CAD build for the part. Positions are in the model's coordinates, mm. Give positions to 0.01 mm unless a question says otherwise; leave off trailing zeros. Write each loop counter-clockwise with the first axis right and the second up, starting at its lowest first coordinate (ties: lowest second). Pieces come first, ordered by that corner, then holes. Notation, with made-up numbers: (-16.75, 25.25) -> (37.25, 25.25) arc R20 ccw to (37.25, 60.25) -> close; hole circle Ø6 at (29.25, 84). An arc over 180 degrees is marked (long way). Answer as a JSON object with one key per item and string values.
```python
from build123d import *

# Parameters (mm, degrees)
ESQUISSE1_R             = 71.6
ESQUISSE1_R_2           = 33.05
BOSS_EXTRU_1_DEPTH      = 5
ESQUISSE2_R             = 6.5
ENL_V_MAT_EXTRU_1_DEPTH = 6
ESQUISSE3_R             = 3.1
ENL_V_MAT_EXTRU_2_DEPTH = 6
CHANFREIN1_SIZE         = 4


with BuildPart() as part:
    # Esquisse1 → Boss.-Extru.1 (new body)
    with BuildSketch(Plane.XY):
        Circle(ESQUISSE1_R)
        Circle(ESQUISSE1_R_2, mode=Mode.SUBTRACT)
    extrude(amount=BOSS_EXTRU_1_DEPTH)

    # Esquisse2 → Enlèv. mat.-Extru.1 (cut, through all)
    with BuildSketch(Plane.XY.offset(5)):
        with Locations((0, 54)):
            Circle(ESQUISSE2_R)
        with Locations((54, 0)):
            Circle(ESQUISSE2_R)
        with Locations((-54, 0)):
            Circle(ESQUISSE2_R)
        with Locations((0, -54)):
            Circle(ESQUISSE2_R)
    extrude(amount=-ENL_V_MAT_EXTRU_1_DEPTH, mode=Mode.SUBTRACT)

    # Esquisse3 → Enlèv. mat.-Extru.2 (cut, through all)
    with BuildSketch(Plane.XY.offset(5)):
        with Locations((-38.183766184, 38.183766184)):
            Circle(ESQUISSE3_R)
        with Locations((38.183766184, -38.183766184)):
            Circle(ESQUISSE3_R)
    extrude(amount=-ENL_V_MAT_EXTRU_2_DEPTH, mode=Mode.SUBTRACT)

    # Chanfrein1
    chanfrein1_edges = [part.edges().sort_by_distance(p)[0] for p in [
        (-41.283766184, 38.183766184, 5),
        (35.083766184, -38.183766184, 5),
    ]]
    chamfer(chanfrein1_edges, length=CHANFREIN1_SIZE)


solid = part.part
```
1) Slice it at C-C (y = 54). List the corners of the cut face in (x, z).
Model answer:
{"outline": "(-47.02, 0) -> (-6.5, 0) -> (-6.5, 5) -> (-47.02, 5) -> close; (6.5, 0) -> (47.02, 0) -> (47.02, 5) -> (6.5, 5) -> close"}
2) Wall check: probe 1 along Y at (x, z) = (0, 3.7); probe 2 along X at (y, z) = (-18.5, 3.7); probe 3 along X at (y, z) = (-52, 2.1). Give the ranges that are in metal, low to high.
Model answer:
{"probe 1": "y = -71.6 to -60.5, -47.5 to -33.05, 33.05 to 47.5, 60.5 to 71.6", "probe 2": "x = -69.17 to -27.39, 27.39 to 69.17", "probe 3": "x = -49.22 to -6.18, 6.18 to 49.22"}
3) Pin check, flat tips, straight feed: pin 1 (5 mm diameter, centred on x = -38.18, y = 38.18, fed in from -Z); pin 2 (2 mm diameter, centred on y = -18.5, z = 1.5, fed in from -X); pin 3 (2 mm diameter, centred on x = -15.5, z = 3.5, fed in from +Y); pin 4 (1 mm diameter, centred on x = 35, z = 1.5, fed in from +Y). Stop position of each tip, or through.
Model answer:
{"pin 1": "passes through", "pin 2": "stops at x = -69.43", "pin 3": "stops at y = 70.12", "pin 4": "stops at y = 62.74"}
4) Mould opens along Y. For faces 1 (the conical face through (-41.47, 38.33, 1.19)), 2 (the cylindrical face through (-47.8, 1.95, 2.54)), 3 (the flat face through (31, -15, 5)), 4 (the cylindrical face through (-56.819, -43.567, 2.465)) say: released by +Y, released by -Y, zero draft, split by the parting line, or undercut.
Model answer:
{"face 1": "undercut", "face 2": "undercut", "face 3": "zero draft", "face 4": "split by the parting line"}
5) Slice it at A-A (y = 0). List the corners of the cut face in (x, z), then the cut area to 4 significant figures.
Model answer:
{"outline": "(-71.6, 0) -> (-60.5, 0) -> (-60.5, 5) -> (-71.6, 5) -> close; (-47.5, 0) -> (-33.05, 0) -> (-33.05, 5) -> (-47.5, 5) -> close; (33.05, 0) -> (47.5, 0) -> (47.5, 5) -> (33.05, 5) -> close; (60.5, 0) -> (71.6, 0) -> (71.6, 5) -> (60.5, 5) -> close", "area": "255.5 mm2"}
